For this review, take the finished solid that the model builds, in its own axes (mm). A direction names the side the tool comes from. Give positions to 0.01 mm unless a question says otherwise; leave off trailing zeros. Write each loop counter-clockwise with the first axis right and the second up, starting at its lowest first coordinate (ties: lowest second). Pieces come first, ordered by that corner, then holes. Notation, with made-up numbers: (2.5, -23) -> (17.5, -23) arc R14 ccw to (17.5, 0) -> close; hole circle Ø7 at (39, -18.5). An arc over 180 degrees is marked (long way). Write item = value, one per line.
```python
from build123d import *

# Parameters (mm, degrees)
SKETCH1_W           = 34.29
SKETCH1_H           = 21.59
SKETCH1_R           = 1.27
SKETCH1_R_2         = 0.508
BOSS_EXTRUDE1_DEPTH = 1.5699994
FILLET1_R           = 2.54
SKETCH2_W           = 7.5
SKETCH2_H           = 15
BOSS_EXTRUDE2_DEPTH = 9
SKETCH3_W           = 4.699
SKETCH3_H           = 6.35
BOSS_EXTRUDE3_DEPTH = 3.175
SKETCH4_W           = 2.667
SKETCH4_H           = 5.842
CUT_EXTRUDE1_DEPTH  = 3.175
SKETCH6_W           = 8.378747874
SKETCH6_H           = 3.102965804
BOSS_EXTRUDE4_DEPTH = 3.81


with BuildPart() as part:
    # Sketch1 → Boss-Extrude1 (new body)
    with BuildSketch(Plane.XY):
        Rectangle(SKETCH1_W, SKETCH1_H)
        with Locations((-14.605, 8.255)):
            Circle(SKETCH1_R, mode=Mode.SUBTRACT)
        with Locations((-14.605, -8.255)):
            Circle(SKETCH1_R, mode=Mode.SUBTRACT)
        with Locations((14.605, -8.255)):
            Circle(SKETCH1_R, mode=Mode.SUBTRACT)
        with Locations((14.605, 8.255)):
            Circle(SKETCH1_R, mode=Mode.SUBTRACT)
        with Locations((-6.169791694, -8.255)):
            Circle(SKETCH1_R_2, mode=Mode.SUBTRACT)
        with Locations((-3.629791694, -8.255)):
            Circle(SKETCH1_R_2, mode=Mode.SUBTRACT)
        with Locations((-1.089791694, -8.255)):
            Circle(SKETCH1_R_2, mode=Mode.SUBTRACT)
    extrude(amount=BOSS_EXTRUDE1_DEPTH)

    # Fillet1
    fillet1_edges = [part.edges().sort_by_distance(p)[0] for p in [
        (17.145, -10.795, 0.7849997),
        (-17.145, -10.795, 0.7849997),
        (-17.145, 10.795, 0.7849997),
        (17.145, 10.795, 0.7849997),
    ]]
    fillet(fillet1_edges, radius=FILLET1_R)

    # Sketch2 → Boss-Extrude2 (add)
    with BuildSketch(Plane.XY.offset(1.5699994)):
        with Locations((-3.219698951, 2.629795429)):
            Rectangle(SKETCH2_W, SKETCH2_H)
    extrude(amount=BOSS_EXTRUDE2_DEPTH)

    # Sketch3 → Boss-Extrude3 (add)
    with BuildSketch(Plane.XY.offset(1.5699994)):
        with Locations((-14.5415, 0)):
            Rectangle(SKETCH3_W, SKETCH3_H)
    extrude(amount=BOSS_EXTRUDE3_DEPTH)

    # Sketch4 → Cut-Extrude1 (cut)
    with BuildSketch(Plane.ZY.offset(16.891)):
        with Locations((3.1574994, 0)):
            Rectangle(SKETCH4_W, SKETCH4_H)
    extrude(amount=-CUT_EXTRUDE1_DEPTH, mode=Mode.SUBTRACT)

    # Sketch6 → Boss-Extrude4 (add, symmetric)
    with BuildSketch(Plane(origin=(0, 0, 0), x_dir=(1, 0, 0), z_dir=(0, 1, 0))):
        with Locations((12.558008878, -3.121482302)):
            Rectangle(SKETCH6_W, SKETCH6_H)
    extrude(amount=BOSS_EXTRUDE4_DEPTH, both=True)


solid = part.part
```
(1) For pin 1 (6 mm diameter, centred on x = -13.5, z = 9, fed in from -Y); pin 2 (1 mm diameter, centred on x = -12.5, y = -1.5, fed in from +Z) (3 decimals); pin 3 (1.6 mm diameter, centred on x = -6.17, y = -8.26, fed in from +Z); pin 4 (1.3 mm diameter, centred on x = -16, z = 3, fed in from +Y) (3 decimals), all flat-tipped, find the tip position at first contact; note any pin that passes through.
Answers below:
pin_1 = through
pin_2 = 4.745
pin_3 = 1.57
pin_4 = 3.175
(2) Take a section at C-C (x = 15.5). Write out the cut boundary in (y, z), plus the area to 3 significant figures.
Answers below:
outline = (-10.63, 0) -> (-9.16, 0) -> (-9.16, 1.57) -> (-10.63, 1.57) -> close; (-7.35, 0) -> (7.35, 0) -> (7.35, 1.57) -> (3.81, 1.57) -> (3.81, 4.67) -> (-3.81, 4.67) -> (-3.81, 1.57) -> (-7.35, 1.57) -> close; (9.16, 0) -> (10.63, 0) -> (10.63, 1.57) -> (9.16, 1.57) -> close
area = 51.4 mm^2
(3) Tool access review of faces 1 (the face through (-15, 0, 4.745)), 2 (the face through (8.369, 0, 3)), 3 (the face through (-15, -3.175, 3)): name each direction out of +Z, -Z, +X, -X, +Y, -Y from which nothing blocks a thin tool from reaching the whole face with its end or side.
Answers below:
face_1 = +Z, -X, +Y, -Y
face_2 = +Z, +Y, -Y
face_3 = +Z, -X, -Y
(4) To check wall thickness, follow probe 1 along X at (y, z) = (2.5, 2.25); probe 2 along Y at (x, z) = (-16, 3.25) (3 decimals); probe 3 along Z at (x, y) = (6, -4.5). State the ranges of each line that lie inside material, in increasing order.
Answers below:
probe_1 = -13.72 to -12.19, -6.97 to 0.53, 8.37 to 16.75
probe_2 = -3.175 to -2.921, 2.921 to 3.175
probe_3 = 0 to 1.57
(5) Take a section at D-D (z = 8). Write out the cut boundary in (x, y), plus the area to 4 significant figures.
Answers below:
outline = (-6.97, -4.87) -> (0.53, -4.87) -> (0.53, 10.13) -> (-6.97, 10.13) -> close
area = 112.5 mm^2
(6) Take a section at B-B (y = 6). Write out the cut boundary in (x, z) (3 decimals).
Answers below:
outline = (-17.145, 0) -> (17.145, 0) -> (17.145, 1.57) -> (0.53, 1.57) -> (0.53, 10.57) -> (-6.97, 10.57) -> (-6.97, 1.57) -> (-17.145, 1.57) -> close
(7) Take a section at A-A (z = 2.75). Write out the cut boundary in (x, y) (3 decimals).
Answers below:
outline = (-16.891, -3.175) -> (-12.192, -3.175) -> (-12.192, 3.175) -> (-16.891, 3.175) -> (-16.891, 2.921) -> (-13.716, 2.921) -> (-13.716, -2.921) -> (-16.891, -2.921) -> close; (-6.97, -4.87) -> (0.53, -4.87) -> (0.53, 10.13) -> (-6.97, 10.13) -> close; (8.369, -3.81) -> (16.747, -3.81) -> (16.747, 3.81) -> (8.369, 3.81) -> close
(8) The part is to be moulded in two halves that separate along X. For faces 4 (the face through (16.38, 10.07, 0.8)), 5 (the face through (13.6, -9.03, 0.77)), 6 (the face through (-13.43, 7.77, 0.77)), 7 (the face through (0, 0, 0)), say which applies: released by +X, released by -X, zero draft, split by the parting line, or undercut.
Answers below:
face_4 = released by +X
face_5 = undercut
face_6 = undercut
face_7 = zero draft
